Autodesk Inventor part; units mm, degrees
ref_plane "YZ Plane" through (0, 0, 0) normal (1, 0, 0) x (0, 1, 0)
ref_plane "XZ Plane" through (0, 0, 0) normal (0, 1, 0) x (-1, 0, 0)
ref_plane "XY Plane" through (0, 0, 0) normal (0, 0, 1) x (1, 0, 0)
sketch "Sketch1" plane through (0, 0, 0) normal (0, 0, 1) x (1, 0, 0)
  line L0 (-262.5, 0) -> (262.5, 0) construction
  line L1 (0, -149.8) -> (0, 149.8) construction
  line L2 (-187.5, 107) -> (187.5, 107)
  line L3 (187.5, 107) -> (187.5, -107)
  line L4 (187.5, -107) -> (-187.5, -107)
  line L5 (-187.5, -107) -> (-187.5, 107)
  point P0 (-167.5, 95)
  point P1 (167.5, 95)
  point P2 (-167.5, -95)
  point P3 (167.5, -95)
  point P4 (0, 0)
  point P5 (-175, 0)
  point P6 (175, 0)
  point P7 (0, -50)
  point P8 (0, 50)
  point P9 (0, 20)
  point P10 (175, 20)
  point P11 (-175, 20)
  dimension "d0" = 375
  dimension "d1" = 214
  dimension "d3" = 335
  dimension "d30" = 20
  dimension "d45" = 12
  dimension "d46" = 190
  dimension "d47" = 100
  dimension "d48" = 12.5
  dimension "d52" = 20
extrude "Extrusion1" add sketch "Sketch1" against normal blind 10
hole "Hole1" at (-167.5, 95, 0) at (167.5, 95, 0) at (-167.5, -95, 0) at (167.5, -95, 0) at (0, -50, 0) at (0, 50, 0) direction (0, 0, -1) diameter 4.5 end through all countersink diameter 10 countersink angle 90
hole "Hole2" at (0, 0, 0) at (0, 20, 0) direction (0, 0, -1) diameter 10.647 end through all
sketch "Sketch2" plane through (0, 0, -10) normal (0, 0, -1) x (-1, 0, 0)
  point P0 (0, 0)
  point P1 (175, 0)
  point P2 (175, 0)
  point P3 (-175, 0)
  point P4 (-175, 0)
  point P5 (0, 20)
  point P6 (0, 0)
  point P7 (175, 20)
  point P8 (-175, 20)
hole "Hole4" at (-175, 0, -10) at (175, 0, -10) at (-175, 20, -10) at (175, 20, -10) direction (0, 0, 1) diameter 6.5 end through all countersink diameter 14.5 countersink angle 90
fillet "Arredondamento2" radius 5 4 edges at (187.5, -107, -5) (187.5, 107, -5) (-187.5, -107, -5) (-187.5, 107, -5)
properties part number "FCT-01-171A" material "Acrílico TP"
Design review of the part built by this model. Coordinates are the model's own, in mm. Coordinates: 2 decimals unless noted, no trailing zeros. Answer as a JSON object with one key per item and string values.
Item 1: Wall thickness on probe 1 along Y at (x, z) = (175, -4.1); probe 2 along X at (y, z) = (-95, -7.5); probe 3 along Y at (x, z) = (0, -7.75): over which ranges is each line inside the solid? List them lowest first.
Outcome:
{"probe 1": "-107 to -3.25, 3.25 to 16.75, 23.25 to 107", "probe 2": "-187.5 to -169.75, -165.25 to 165.25, 169.75 to 187.5", "probe 3": "-107 to -52.25, -47.75 to -5.32, 5.32 to 14.68, 25.32 to 47.75, 52.25 to 107"}
Item 2: Insertion check: pin 1 Ø5 at (x, y) = (-175, 20) entering from -Z; pin 2 Ø7.5 at (x, y) = (-175, 0) entering from -Z; pin 3 Ø7 at (x, y) = (167.5, -95) entering from +Z; pin 4 Ø8.5 at (x, y) = (175, 0) entering from +Z. Each pin has a flat end and moves straight along its axis. Give the tip position at first contact, or say it passes through.
Outcome:
{"pin 1": "through", "pin 2": "z = -6.5", "pin 3": "z = -1.5", "pin 4": "z = 0"}
Item 3: Draft analysis for pull direction X (two halves, no side actions). For faces 1 (the flat face through (-3, 107, -5)), 2 (the flat face through (187.5, 1, -5)), 3 (the conical face through (171.895, 21.615, -6.25)), state which applies: pulls with the +X half, pulls with the -X half, needs draft (parallel to the pull), parting line crosses it, or undercut.
Outcome:
{"face 1": "needs draft", "face 2": "pulls with the +X half", "face 3": "undercut"}
